Solid Edge part; units mm, degrees
sketch "Sketch1" plane through (0, 0, 0) normal (0, -1, 0) x (1, 0, 0)
  arc A0 (7.2243, 1.8396) -> (8.2243, 2.8396) centre (7.2243, 2.8396) ccw
  line L0 (8.2243, 2.8396) -> (8.2243, 3.3396)
  arc A1 (8.2243, 3.3396) -> (7.2243, 4.3396) centre (7.2243, 3.3396) ccw
  line L1 (7.2243, 4.3396) -> (5.2243, 4.3396)
  arc A2 (4.2243, 3.3396) -> (5.2243, 4.3396) centre (5.2243, 3.3396) cw
  line L2 (4.2243, 3.3396) -> (4.2243, 2.8396)
  arc A3 (4.2243, 2.8396) -> (5.2243, 1.8396) centre (5.2243, 2.8396) ccw
  line L3 (5.2243, 1.8396) -> (7.2243, 1.8396)
revolve "RevolvedProtrusion1" add sketch "Sketch1" angle 360 about axis through (6.2243, 0, -31.6604) along (1, 0, 0)
Could you check a few things on this model? Use its own coordinates, in mm. Coordinates: 2 decimals unless noted, no trailing zeros. Loops run counter-clockwise (first coordinate to the right, second up) from the corner with the lowest first, then second, coordinate; pieces in that order, holes last. Notation, with made-up numbers: M 44,-23.75 L 69,-23.75 A18 cw 69,4.25 Z; hole C 19,-36 d9. An arc over 180 degrees is marked long. Put each result on its own line as item: value. Start each with the question number.
(1) I need wall thicknesses on line 1 (Z direction, x = 6.05, y = 0); line 2 (Z direction, x = 4.4, y = 17); line 3 (Y direction, x = 4.8, z = -43.5). Which ranges of each line are inside material? Lowest first, please. Write a range as from..to.
(2) Will these pins go through, and if not, where does the flat tip stop? P1, Ø2, axis at x = 5, z = -26, coming from the +Y side; P2, Ø1.5, axis at x = 5, y = -10, coming from the -Z side; P3, Ø1, axis at x = 7.5, y = -22, coming from the +Z side.
(3) Thinking about a two-plate mould opening in Z: for faces 1 (the face through (4.224, 23.2, -5.9)), 2 (the face through (6.238, -10.062, 0.293)), 3 (the face through (6.21, 10.81, 2.68)), which applies, pulls with the +Z half, pulls with the -Z half, needs draft (parallel to the pull), parting line crosses it, or undercut?
(4) Suppose I cut it at A-A on y = 0. Please give me the cut outline in (x, z), then the cut area to 3 significant figures.
(5) Suppose I cut it at B-B on x = 5.9. Please give me the cut outline in (y, z).
Solutions:
1. line 1: z = -67.66..-65.16, 1.84..4.34
1. line 2: z = -62.9..-61.03, -2.29..-0.42
1. line 3: y = -33.9..-31.44, 31.44..33.9
2. P1: stops at y = 35.69
2. P2: stops at z = -66.45
2. P3: stops at z = -2.81
3. face 1: needs draft
3. face 2: undercut
3. face 3: parting line crosses it
4. outline: M 4.22,-66.66 A1 ccw 5.22,-67.66 L 7.22,-67.66 A1 ccw 8.22,-66.66 L 8.22,-66.16 A1 ccw 7.22,-65.16 L 5.22,-65.16 A1 ccw 4.22,-66.16 Z; M 4.22,2.84 A1 ccw 5.22,1.84 L 7.22,1.84 A1 ccw 8.22,2.84 L 8.22,3.34 A1 ccw 7.22,4.34 L 5.22,4.34 A1 ccw 4.22,3.34 Z
4. area: 18.3 mm2
5. outline: C 0,-31.66 d72; hole C 0,-31.66 d67
